Geometry: see drawing. Coordinates: mm, zero at the bounding-box minimum. Coordinates: 2 decimals unless noted, no trailing zeros. Loops run counter-clockwise (first coordinate to the right, second up) from the corner with the lowest first, then second, coordinate; pieces in that order, holes last. Notation, with made-up numbers: (85, 54.25) - (126, 54.25) arc R22 ccw to (126, 84.25) - close; hole circle Ø3 at (-16.75, 21.5). An arc over 180 degrees is marked (long way). Answer in a Markdown table with one row per item.
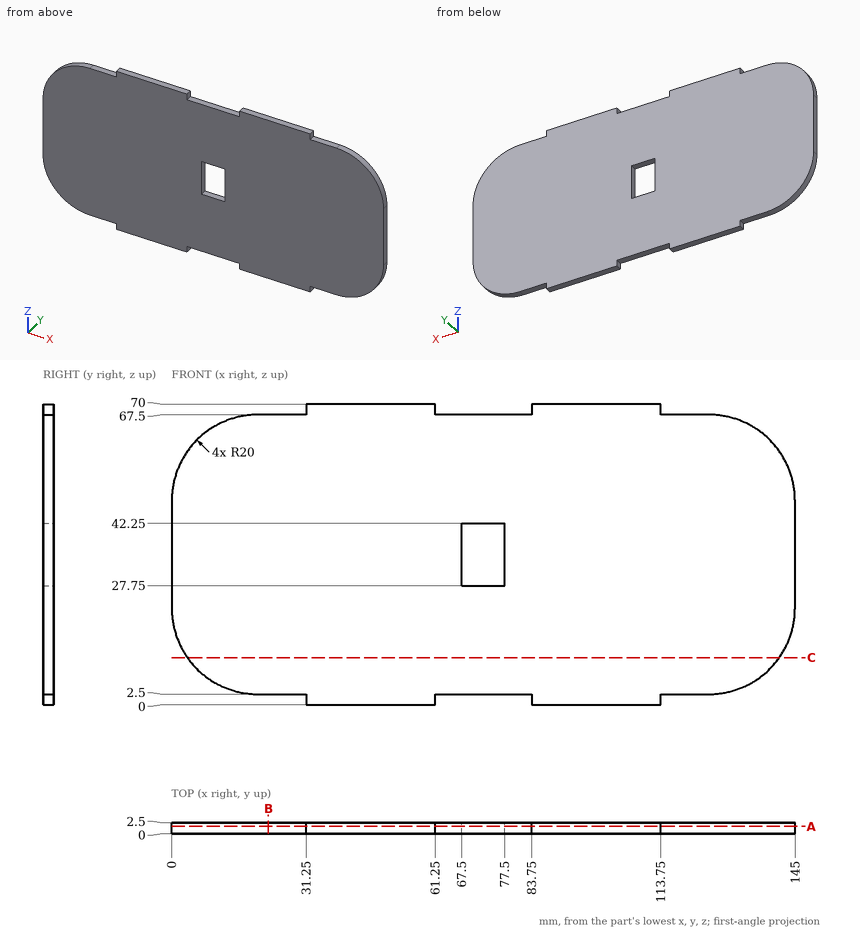
(1) Cut plane C-C on z = 11. Output: boundary loops of the cut face in (x, y).
Verdict:
| item | result |
|---|---|
| outline | (3.64, 0) - (141.36, 0) - (141.36, 2.5) - (3.64, 2.5) - close |
(2) First-contact query: pin 1 Ø1 at (y, z) = (1, 53) entering from +X; pin 2 Ø0.8 at (x, y) = (23, 1) entering from +Z; pin 3 Ø0.8 at (y, z) = (1, 69) entering from +X; pin 4 Ø6 at (x, z) = (125, 23) entering from -Y. Flat tips, straight axial feed; report the tip coordinate or a pass-through.
Verdict:
| item | result |
|---|---|
| pin 1 | stops at x = 144.36 |
| pin 2 | stops at z = 67.5 |
| pin 3 | stops at x = 113.75 |
| pin 4 | stops at y = 0 |
(3) Cut plane B-B on x = 22.5. Output: boundary loops of the cut face in (y, z).
Verdict:
| item | result |
|---|---|
| outline | (0, 2.5) - (2.5, 2.5) - (2.5, 67.5) - (0, 67.5) - close |
(4) Cut plane A-A on y = 1.7. Output: boundary loops of the cut face in (x, z).
Verdict:
| item | result |
|---|---|
| outline | (0, 22.5) arc R20 ccw to (20, 2.5) - (31.25, 2.5) - (31.25, 0) - (61.25, 0) - (61.25, 2.5) - (83.75, 2.5) - (83.75, 0) - (113.75, 0) - (113.75, 2.5) - (125, 2.5) arc R20 ccw to (145, 22.5) - (145, 47.5) arc R20 ccw to (125, 67.5) - (113.75, 67.5) - (113.75, 70) - (83.75, 70) - (83.75, 67.5) - (61.25, 67.5) - (61.25, 70) - (31.25, 70) - (31.25, 67.5) - (20, 67.5) arc R20 ccw to (0, 47.5) - close; hole (67.5, 27.75) - (77.5, 27.75) - (77.5, 42.25) - (67.5, 42.25) - close |
(5) Ray query, probe 1 along X at (y, z) = (0.2, 29.5); probe 2 along Z at (x, y) = (125, 1.2); probe 3 along X at (y, z) = (1.05, 16.5). Return the intervals inside material, ascending.
Verdict:
| item | result |
|---|---|
| probe 1 | x = 0 to 67.5, 77.5 to 145 |
| probe 2 | z = 2.5 to 67.5 |
| probe 3 | x = 0.92 to 144.08 |
